Geometry check sheet. Reference: the model listing, model coordinates, mm. A direction names the side the tool comes from. Round coordinates to 2 decimals unless told otherwise and drop trailing zeros. Order: outer loops, then holes, each group sorted by start corner. A loop starts at its lowest first (then second) coordinate and runs counter-clockwise, first axis right, second up.
(1) Material ranges on line 1 along Y through (x, z) = (8.25, 0.1); line 2 along X through (y, z) = (-1, 2.2), recorded low to high.
(2) Release check for a two-part mould opening along Y. For faces 4 (the face through (-2.408, -0.491, 0.867)), 5 (the face through (-3, 1, -1)), 6 (the face through (-1.482, -0.596, -2.685)) record: +Y half, -Y half, draft (parallel to the pull), parting line (faces both ways), or undercut.
(3) Sectioned sample at B-B (z = 0). Record the boundary of the cut face in (x, y), plus the area to 3 significant figures.
(4) Sectioned sample at A-A (x = -2). Record the boundary of the cut face in (y, z) (3 decimals).
(5) Set-up check for faces 1 (the face through (12, 0, 0)), 2 (the face through (0, 2, 0)), 3 (the face through (-2, -0.996, 0)): record each of +Z, -Z, +X, -X, +Y, -Y from which the full face is reachable in a straight line by a thin tool's end or side.
(6) Go/stop test with flat-tipped pins: pin 1 (3 mm diameter, centred on x = 2.5, z = 2, fed in from +Y); pin 2 (2 mm diameter, centred on x = 10, y = 1, fed in from -Z). Record where each tip stops, or that it passes through.
(7) Sectioned sample at C-C (x = 6.5). Record the boundary of the cut face in (y, z).
Autodesk Inventor part; units mm, degrees
ref_plane "YZ Plane" through (0, 0, 0) normal (1, 0, 0) x (0, 1, 0)
ref_plane "XZ Plane" through (0, 0, 0) normal (0, 1, 0) x (-1, 0, 0)
ref_plane "XY Plane" through (0, 0, 0) normal (0, 0, 1) x (1, 0, 0)
sketch "スケッチ1" plane through (0, 0, 0) normal (0, 0, 1) x (1, 0, 0)
  line L0 (0, 0) -> (12, 0)
  line L1 (12, 0) -> (12, 1.5)
  line L2 (12, 1.5) -> (0, 1.5)
  line L3 (0, 1.5) -> (0, 0)
  line L4 (0, 0) -> (0, 2.75)
  line L5 (0, 0) -> (-3, 0)
  line L6 (-3, 0) -> (0, 0)
  line L7 (-3, 0) -> (-3, 1.15)
  line L8 (0, 0) -> (-3, 0)
  line L9 (-3, 0) -> (-3, 2.75)
  line L10 (-3, 2.75) -> (0, 2.75)
  line L11 (0, 2.75) -> (0, 0)
  dimension "d0" = 1.5
  dimension "d1" = 12
  dimension "d3" = 3
  dimension "d4" = 2.75
  dimension "d5" = 1.15
revolve "回転1" add sketch "スケッチ1" angle 360 about axis through (-3, 0, 0) along (1, 0, 0)
thread "ねじ1"
sketch "スケッチ2" plane through (-3, 0, 0) normal (-1, 0, 0) x (0, 0, 1)
  circle A0 centre (0, 0) radius 1.15
  line L0 (-0.575, 0.9959) -> (0.575, 0.9959)
  line L1 (0.575, 0.9959) -> (1.15, 0)
  line L2 (1.15, 0) -> (0.575, -0.9959)
  line L3 (0.575, -0.9959) -> (-0.575, -0.9959)
  line L4 (-0.575, -0.9959) -> (-1.15, 0)
  line L5 (-1.15, 0) -> (-0.575, 0.9959)
  dimension "d10" = 1.15
  dimension "d11" = 1.9919
extrude "押し出し1" cut sketch "スケッチ2" against normal blind 1.4 contours L2 L3 L4 L5 L0 L1
fillet "フィレット1" radius 0.2 8 edges at (-1.6, 0.9959, 0) (-1.6, 0.498, 0.8625) (-1.6, 0.498, -0.8625) (-1.6, -0.498, -0.8625) (-1.6, -0.9959, 0) (-1.6, -0.498, 0.8625) (-3, -2.75, 0) (0, -2.75, 0)
fillet "フィレット2" radius 0.1 1 edges at (0, -1.5, 0)
fillet "フィレット3" radius 0.1 1 edges at (12, -1.5, 0)
properties part number "ネジアルミM3L122" material "アルミニウム 7075"
Answer below:
1. line 1: y = -1.5 to 1.5
1. line 2: x = -3 to 0
2. face 4: undercut
2. face 5: draft
2. face 6: parting line
3. outline: (-3, -2.55) arc R0.2 ccw to (-2.8, -2.75) - (-0.2, -2.75) arc R0.2 ccw to (0, -2.55) - (0, -1.6) arc R0.1 cw to (0.1, -1.5) - (11.9, -1.5) arc R0.1 ccw to (12, -1.4) - (12, 1.4) arc R0.1 ccw to (11.9, 1.5) - (0.1, 1.5) arc R0.1 cw to (0, 1.6) - (0, 2.55) arc R0.2 ccw to (-0.2, 2.75) - (-2.8, 2.75) arc R0.2 ccw to (-3, 2.55) - (-3, 1) - (-1.8, 1) arc R0.2 cw to (-1.6, 0.8) - (-1.6, -0.8) arc R0.2 cw to (-1.8, -1) - (-3, -1) - close
3. area: 49.7 mm2
4. outline: circle Ø5.5 at (0, 0); hole (-0.996, -0.575) - (0, -1.15) - (0.996, -0.575) - (0.996, 0.575) - (0, 1.15) - (-0.996, 0.575) - close
5. face 1: +Z, -Z, +X, +Y, -Y
5. face 2: +X
5. face 3: -X
6. pin 1: stops at y = 1.41
6. pin 2: stops at z = -1.5
7. outline: circle Ø3 at (0, 0)
